The model under review builds one solid part; all positions refer to its coordinate system, in mm. A direction names the side the tool comes from. Coordinates: 2 decimals unless noted, no trailing zeros. Order: outer loops, then holes, each group sorted by start corner. A loop starts at its lowest first (then second) coordinate and runs counter-clockwise, first axis right, second up. Notation, with made-up numbers: (-27, 70) -> (-19, 70) arc R24 cw to (-19, 93) -> close; hole circle Ø10 at (-12.5, 88). An arc over 180 degrees is marked (long way). Use one line per item in the form item = value.
from build123d import *

# Parameters (mm, degrees)
SKETCH_W        = 178
SKETCH_H        = 88
PAD_DEPTH       = 74
SKETCH001_W     = 170
SKETCH001_H     = 80
POCKET_DEPTH    = 70
SKETCH002_W     = 12.5
SKETCH002_H     = 11
SKETCH002_W_2   = 9.5
SKETCH002_H_2   = 11.5
POCKET001_DEPTH = 5
SKETCH003_W     = 30
SKETCH003_H     = 30
POCKET002_DEPTH = 5
SKETCH004_W     = 13
SKETCH004_H     = 19
POCKET003_DEPTH = 5
SKETCH005_R     = 4.5
POCKET004_DEPTH = 5
SKETCH006_W     = 6
SKETCH006_H     = 6.5
PAD001_DEPTH    = 30
SKETCH007_R     = 4.5
POCKET005_DEPTH = 90
SKETCH008_R     = 1.55
PAD002_DEPTH    = 3
SKETCH010_R     = 1.75
POCKET006_DEPTH = 5
SKETCH011_W     = 4
SKETCH011_H     = 4
PAD004_DEPTH    = 6


with BuildPart() as part:
    # Sketch → Pad (new body)
    with BuildSketch(Plane.XY):
        with Locations((89, 44)):
            Rectangle(SKETCH_W, SKETCH_H)
    extrude(amount=PAD_DEPTH)

    # Sketch001 (on Face6 of Pad) → Pocket (cut)
    with BuildSketch(Plane.XY.offset(74)):
        with Locations((89, 44)):
            Rectangle(SKETCH001_W, SKETCH001_H)
    extrude(amount=-POCKET_DEPTH, mode=Mode.SUBTRACT)

    # Sketch002 (on Face3 of Pocket) → Pocket001 (cut)
    with BuildSketch(Plane.YZ.offset(178)):
        with Locations((21.25, 13.5)):
            Rectangle(SKETCH002_W, SKETCH002_H)
        with Locations((52.25, 13.75)):
            Rectangle(SKETCH002_W_2, SKETCH002_H_2)
    extrude(amount=-POCKET001_DEPTH, mode=Mode.SUBTRACT)

    # Sketch003 (on Face3 of Pocket001) → Pocket002 (cut)
    with BuildSketch(Plane.YZ.offset(178)):
        with Locations((44, 45)):
            Rectangle(SKETCH003_W, SKETCH003_H)
    extrude(amount=-POCKET002_DEPTH, mode=Mode.SUBTRACT)

    # Sketch004 (on Face1 of Pocket002) → Pocket003 (cut)
    with BuildSketch(Plane.XZ):
        with Locations((136.5, 30.5)):
            Rectangle(SKETCH004_W, SKETCH004_H)
    extrude(amount=-POCKET003_DEPTH, mode=Mode.SUBTRACT)

    # Sketch005 (on Face2 of Pocket003) → Pocket004 (cut)
    with BuildSketch(Plane(origin=(0, 0, 0), x_dir=(0, -1, 0), z_dir=(-1, 0, 0))):
        with Locations((-67, 34)):
            Circle(SKETCH005_R)
    extrude(amount=-POCKET004_DEPTH, mode=Mode.SUBTRACT)

    # Sketch006 (on Face28 of Pocket004) → Pad001 (join)
    with BuildSketch(Plane.XY.offset(4)):
        with Locations((32, 67)):
            Rectangle(SKETCH006_W, SKETCH006_H)
        with Locations((55, 67)):
            Rectangle(SKETCH006_W, SKETCH006_H)
        with Locations((75, 67)):
            Rectangle(SKETCH006_W, SKETCH006_H)
    extrude(amount=PAD001_DEPTH)

    # Sketch007 (on Face31 of Pad001) → Pocket005 (cut)
    with BuildSketch(Plane.YZ.offset(78)):
        with Locations((67, 34)):
            Circle(SKETCH007_R)
    extrude(amount=-POCKET005_DEPTH, mode=Mode.SUBTRACT)

    # Sketch008 (on Face29 of Pocket005) → Pad002 (join)
    with BuildSketch(Plane.XY.offset(4)):
        with Locations((104.96, 52)):
            Circle(SKETCH008_R)
        with Locations((104.96, 24)):
            Circle(SKETCH008_R)
    extrude(amount=PAD002_DEPTH)

    # Sketch010 → Pocket006 (cut)
    with BuildSketch(Plane.YZ.offset(178)):
        with Locations((70, 10)):
            Circle(SKETCH010_R)
    extrude(amount=-POCKET006_DEPTH, mode=Mode.SUBTRACT)

    # Sketch011 (on Face30 of Pocket006) → Pad004 (join)
    with BuildSketch(Plane.XY.offset(4)):
        with Locations((10, 31)):
            Rectangle(SKETCH011_W, SKETCH011_H)
        with Locations((20, 64)):
            Rectangle(SKETCH011_W, SKETCH011_H)
        with Locations((101, 15)):
            Rectangle(SKETCH011_W, SKETCH011_H)
        with Locations((92, 64)):
            Rectangle(SKETCH011_W, SKETCH011_H)
    extrude(amount=PAD004_DEPTH)


solid = part.part
Item 1: We need section B-B (y = 37). Write out the cut boundary in (x, z), plus the area to 3 significant figures.
Results found:
outline = (0, 0) -> (178, 0) -> (178, 30) -> (174, 30) -> (174, 4) -> (4, 4) -> (4, 74) -> (0, 74) -> close; (174, 60) -> (178, 60) -> (178, 74) -> (174, 74) -> close
area = 1,150 mm²
Item 2: We need section D-D (x = 68.5). Write out the cut boundary in (y, z), plus the area to 3 significant figures.
Results found:
outline = (0, 0) -> (88, 0) -> (88, 74) -> (84, 74) -> (84, 4) -> (4, 4) -> (4, 74) -> (0, 74) -> close
area = 912 mm²
Item 3: Draft analysis for pull direction Z (two halves, no side actions). For faces 1 (the face through (88, 84, 39)), 2 (the face through (55, 66.9, 29.5)), 3 (the face through (176, 57, 14)), state which applies: released by +Z, released by -Z, zero draft, split by the parting line, or undercut.
Results found:
face_1 = zero draft
face_2 = released by +Z
face_3 = undercut
Item 4: We need section A-A (z = 34). Write out the cut boundary in (x, y).
Results found:
outline = (0, 0) -> (130, 0) -> (130, 4) -> (4, 4) -> (4, 62.5) -> (0, 62.5) -> close; (0, 71.5) -> (4, 71.5) -> (4, 84) -> (174, 84) -> (174, 59) -> (178, 59) -> (178, 88) -> (0, 88) -> close; (143, 0) -> (178, 0) -> (178, 29) -> (174, 29) -> (174, 4) -> (143, 4) -> close
Item 5: Clearance check with a flat-ended pin moving along its axis: pin 1 (2 mm diameter, centred on y = 55, z = 36, fed in from +X). State where the tip first meets the part, or that it passes through.
Results found:
pin_1 = 4
Item 6: To check wall thickness, follow L1, parallel to Y at x = 53, z = 12; L2, parallel to X at y = 12.5, z = 32; L3, parallel to Y at x = 68, z = 6. State the ranges of each line that lie inside material, in increasing order. Write a range as from..to.
Results found:
L1 = 0..4, 63.75..70.25, 84..88
L2 = 0..4, 174..178
L3 = 0..4, 84..88
Item 7: Tool access review of faces 4 (the face through (136, 2, 21)), 5 (the face through (8, 31, 7)), 6 (the face through (176, 44, 60)), 7 (the face through (88, 0, 36)): name each direction out of +Z, -Z, +X, -X, +Y, -Y from which nothing blocks a thin tool from reaching the whole face with its end or side.
Results found:
face_4 = -Y
face_5 = +Z
face_6 = +X
face_7 = +Z, -Z, +X, -X, -Y
Item 8: We need section C-C (z = 23). Write out the cut boundary in (x, y).
Results found:
outline = (0, 0) -> (130, 0) -> (130, 4) -> (4, 4) -> (4, 84) -> (174, 84) -> (174, 4) -> (143, 4) -> (143, 0) -> (178, 0) -> (178, 88) -> (0, 88) -> close; (29, 63.75) -> (35, 63.75) -> (35, 70.25) -> (29, 70.25) -> close; (52, 63.75) -> (58, 63.75) -> (58, 70.25) -> (52, 70.25) -> close; (72, 63.75) -> (78, 63.75) -> (78, 70.25) -> (72, 70.25) -> close
